from build123d import *

# Parameters (mm, degrees)
F1_DEPTH = 25.4
F2_R     = 3.170865
F3_DEPTH = 25.401
F4_R     = 1.5875
F5_DEPTH = 3.175


with BuildPart() as f1:
    # F0 (on Right) → F1 (new body)
    with BuildSketch(Plane.YZ):
        Polygon((-168.275, -12.7), (142.875, -12.7), (142.875, -19.05), (168.275, -19.05), (168.275, -12.7), (168.275, 12.7), (168.275, 38.1), (142.875, 38.1), (142.875, 12.7), (-168.275, 12.7), align=None)
    extrude(amount=F1_DEPTH)

    # F2 (on face) → F3 (cut, through all)
    with BuildSketch(Plane.YZ.offset(25.4)):
        with Locations((-139.785126, 0)):
            Circle(F2_R)
    extrude(amount=-F3_DEPTH, mode=Mode.SUBTRACT)

    # F4 (on face) → F5 (cut)
    with BuildSketch(Plane.XY.offset(12.7)):
        with Locations((12.7, 139.7)):
            Circle(F4_R)
    extrude(amount=-F5_DEPTH, mode=Mode.SUBTRACT)


solid = f1.part
Verification items for the finished model (mm, model axes). A direction names the side the tool comes from. Give positions to 0.01 mm unless a question says otherwise; leave off trailing zeros. Write each loop counter-clockwise with the first axis right and the second up, starting at its lowest first coordinate (ties: lowest second). Pieces come first, ordered by that corner, then holes. Notation, with made-up numbers: (77.25, 44.5) -> (91.25, 44.5) arc R25 cw to (91.25, 69.5) -> close; hole circle Ø8 at (59.25, -39.5). An arc over 180 degrees is marked (long way). Use CSV: the item, a comma, the result in double quotes.
(1) Sectioned sample at A-A (x = 4.25). Record the cut outline in (y, z) (3 decimals).
Derived:
outline,"(-168.275, -12.7) -> (142.875, -12.7) -> (142.875, -19.05) -> (168.275, -19.05) -> (168.275, 38.1) -> (142.875, 38.1) -> (142.875, 12.7) -> (-168.275, 12.7) -> close; hole circle Ø6.342 at (-139.785, 0)"
(2) Sectioned sample at C-C (y = -146). Record the cut outline in (x, z).
Derived:
outline,"(0, -12.7) -> (25.4, -12.7) -> (25.4, 12.7) -> (0, 12.7) -> close"
(3) Set-up check for faces 4 (the flat face through (0, -2, 4)), 5 (the flat face through (13, -11, 12.7)), 6 (the flat face through (13, 142.875, -16)): record each of +Z, -Z, +X, -X, +Y, -Y from which the full face is reachable in a straight line by a thin tool's end or side.
Derived:
face 4,"+Z, -Z, -X, +Y, -Y"
face 5,"+Z, +X, -X, -Y"
face 6,"-Z, +X, -X, -Y"
(4) Material ranges on L1, parallel to Y at x = 12.7, z = 10.9 (1 decimal); L2, parallel to X at y = 139.7, z = 10.4; L3, parallel to Z at x = 17, y = -130.5, recorded low to high.
Derived:
L1,"y = -168.3 to 138.1, 141.3 to 168.3"
L2,"x = 0 to 11.11, 14.29 to 25.4"
L3,"z = -12.7 to 12.7"
(5) Release check for a two-part mould opening along Y. For faces 1 (the flat face through (13, 142.875, 26)), 2 (the cylindrical face through (12.878, -136.856, -1.214)), 3 (the flat face through (13, -15, -12.7)) record: +Y half, -Y half, draft (parallel to the pull), parting line (faces both ways), or undercut.
Derived:
face 1,"-Y half"
face 2,"undercut"
face 3,"draft"
(6) Sectioned sample at B-B (z = 0). Record the cut outline in (x, y) (3 decimals).
Derived:
outline,"(0, -168.275) -> (25.4, -168.275) -> (25.4, -142.956) -> (0, -142.956) -> close; (0, -136.614) -> (25.4, -136.614) -> (25.4, 168.275) -> (0, 168.275) -> close"
(7) Go/stop test with flat-tipped pins: pin 1 (1.6 mm diameter, centred on x = 12, y = 139.5, fed in from +Z) (3 decimals); pin 2 (1 mm diameter, centred on x = 17, y = -41, fed in from +Z); pin 3 (7.5 mm diameter, centred on x = 10.5, z = 29.5, fed in from -Y) (3 decimals). Record where each tip stops, or that it passes through.
Derived:
pin 1,"stops at z = 9.525"
pin 2,"stops at z = 12.7"
pin 3,"stops at y = 142.875"
